Part print with two shaded views. Sizes in mm from the minimum x, y, z corner. Round coordinates to 2 decimals unless told otherwise and drop trailing zeros. Order: outer loops, then holes, each group sorted by start corner. A loop starts at its lowest first (then second) coordinate and runs counter-clockwise, first axis right, second up. Notation, with made-up numbers: (48, -4) - (91, -4) arc R24 ccw to (91, 22) - close; hole circle Ø10 at (-21.5, 61). An arc over 180 degrees is marked (long way). Use one line per item in the form item = value.
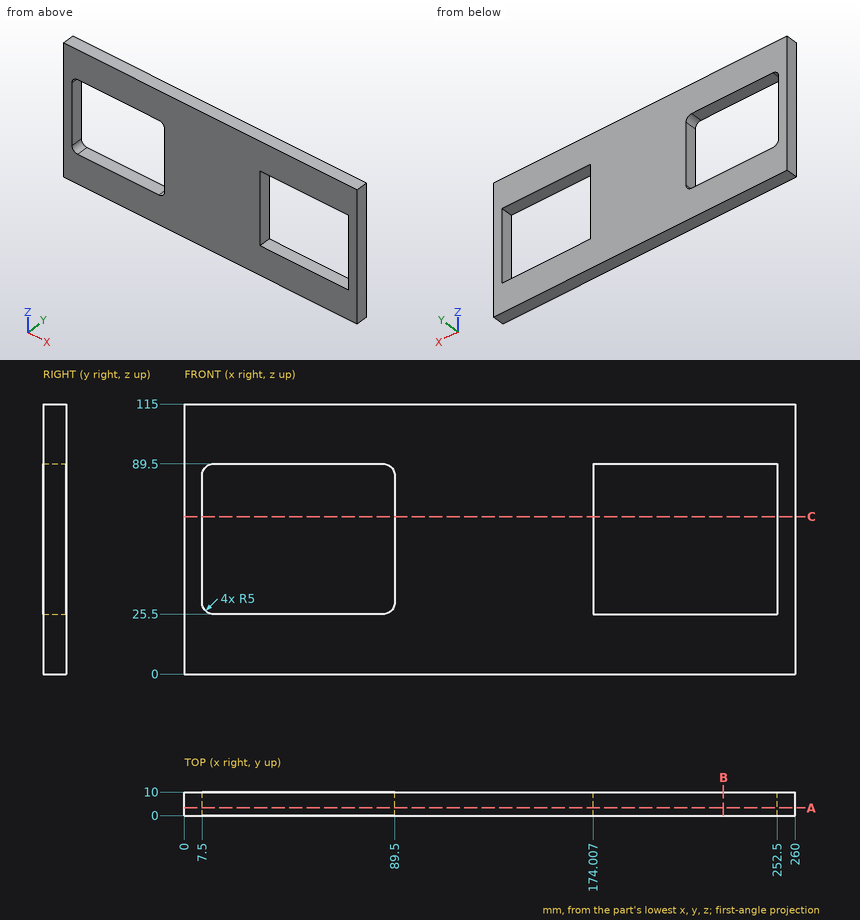
(1) Probe probe 1 along X at (y, z) = (8.5, 57); probe 2 along Z at (x, y) = (220, 7). List the from-to ranges inside material, lowest first. Write a range as [from, to].
Report:
probe_1 = [0, 7.5], [89.5, 174.01], [252.5, 260]
probe_2 = [0, 25.5], [89.5, 115]
(2) Slice it at A-A on y = 3.25. Give the cut face in (x, z).
Report:
outline = (0, 0) - (260, 0) - (260, 115) - (0, 115) - close; hole (7.5, 30.5) arc R5 ccw to (12.5, 25.5) - (84.5, 25.5) arc R5 ccw to (89.5, 30.5) - (89.5, 84.5) arc R5 ccw to (84.5, 89.5) - (12.5, 89.5) arc R5 ccw to (7.5, 84.5) - close; hole (174.01, 25.5) - (252.5, 25.5) - (252.5, 89.5) - (174.01, 89.5) - close
(3) Slice it at C-C on z = 67. Give the cut face in (x, y), then the cut area to 3 significant figures.
Report:
outline = (0, 0) - (7.5, 0) - (7.5, 10) - (0, 10) - close; (89.5, 0) - (174.01, 0) - (174.01, 10) - (89.5, 10) - close; (252.5, 0) - (260, 0) - (260, 10) - (252.5, 10) - close
area = 995 mm2
(4) Slice it at B-B on x = 229.5. Give the cut face in (y, z), then the cut area to 3 significant figures.
Report:
outline = (0, 0) - (10, 0) - (10, 25.5) - (0, 25.5) - close; (0, 89.5) - (10, 89.5) - (10, 115) - (0, 115) - close
area = 510 mm2
